```python
from build123d import *

# Parameters (mm, degrees)
SKETCH1_W               = 20
SKETCH1_H               = 20
BOSS_EXTRUDE1_DEPTH     = 20
CUT_EXTRUDE1_DEPTH      = 1
CUT_EXTRUDE1_DEPTH_BACK = 21
SKETCH3_R               = 3
CUT_EXTRUDE2_DEPTH      = 21
SKETCH4_R               = 3
CUT_EXTRUDE3_DEPTH      = 21
SKETCH5_W               = 15
SKETCH5_H               = 15
CUT_EXTRUDE5_DEPTH      = 17.5
FILLET1_R               = 0.5


with BuildPart() as part:
    # Sketch1 → Boss-Extrude1 (new body)
    with BuildSketch(Plane(origin=(0, 0, 0), x_dir=(1, 0, 0), z_dir=(0, 1, 0))):
        Rectangle(SKETCH1_W, SKETCH1_H)
    extrude(amount=BOSS_EXTRUDE1_DEPTH)

    # Sketch2 → Cut-Extrude1 (cut, two sides)
    with BuildSketch(Plane.XY.offset(10)) as cut_extrude1_sk:
        Polygon((-10, 0), (10, 20), (-10, 20), align=None)
    extrude(amount=CUT_EXTRUDE1_DEPTH, mode=Mode.SUBTRACT)
    extrude(cut_extrude1_sk.sketch, amount=-CUT_EXTRUDE1_DEPTH_BACK, mode=Mode.SUBTRACT)

    # Sketch3 → Cut-Extrude2 (cut, through all)
    with BuildSketch(Plane(origin=(10, 0, 0), x_dir=(0, 0, -1), z_dir=(1, 0, 0))):
        with Locations((0, 10)):
            Circle(SKETCH3_R)
    extrude(amount=-CUT_EXTRUDE2_DEPTH, mode=Mode.SUBTRACT)

    # Sketch4 → Cut-Extrude3 (cut, through all)
    with BuildSketch(Plane.XZ):
        Circle(SKETCH4_R)
    extrude(amount=-CUT_EXTRUDE3_DEPTH, mode=Mode.SUBTRACT)

    # Sketch5 → Cut-Extrude5 (cut)
    with BuildSketch(Plane(origin=(0, 20, 0), x_dir=(1, 0, 0), z_dir=(0, 1, 0))):
        Rectangle(SKETCH5_W, SKETCH5_H)
    extrude(amount=-CUT_EXTRUDE5_DEPTH, mode=Mode.SUBTRACT)

    # Fillet1
    fillet1_edges = [part.edges().sort_by_distance(p)[0] for p in [
        (10, 20, 0),
        (-10, 0, 0),
        (10, 0, 0),
    ]]
    fillet(fillet1_edges, radius=FILLET1_R)


solid = part.part
```
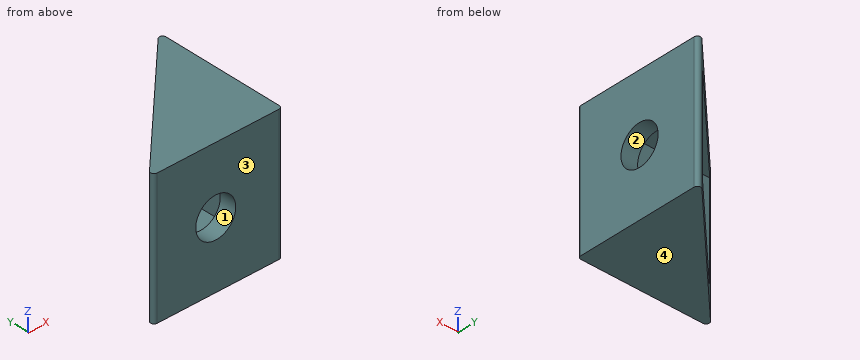
Read the model definition and answer for the solid it produces. Units are mm, in the model's axes. Face numbers are marked on the shaded views. Coordinates: 2 decimals unless noted, no trailing zeros. Write each loop counter-clockwise with the first axis right and the second up, starting at its lowest first coordinate (ties: lowest second). Pieces come first, ordered by that corner, then holes. Notation, with made-up numbers: (43, 74) -> (52, 74) arc R29 ccw to (52, 94) -> close; hole circle Ø4 at (72, 63). An arc over 180 degrees is marked (long way). Answer as a JSON object with one key per item and string values.
Q1. The part is cut by section B-B on z = 0. Give the vertices of the cut face in (x, y), then the cut area to 3 significant figures.
The answers:
{"outline": "(-9.15, 0.85) arc R0.5 ccw to (-8.79, 0) -> (-3, 0) -> (-3, 2.5) -> (-7.5, 2.5) -> close; (3, 0) -> (9.5, 0) arc R0.5 ccw to (10, 0.5) -> (10, 7) -> (7.5, 7) -> (7.5, 2.5) -> (3, 2.5) -> close; (7.5, 13) -> (10, 13) -> (10, 18.79) arc R0.5 ccw to (9.15, 19.15) -> (7.5, 17.5) -> close", "area": "56.8 mm2"}
Q2. The part is cut by section C-C on y = 10. Give the vertices of the cut face in (x, z).
The answers:
{"outline": "(0, -10) -> (10, -10) -> (10, -3) -> (7.5, -3) -> (7.5, -7.5) -> (0, -7.5) -> close; (0, 7.5) -> (7.5, 7.5) -> (7.5, 3) -> (10, 3) -> (10, 10) -> (0, 10) -> close"}
Q3. Determine the mould class of the marked faces 1, 2, 3 and 4 for opening direction Z: pulls with the +Z half, pulls with the -Z half, needs draft (parallel to the pull), parting line crosses it, or undercut.
The answers:
{"face 1": "undercut", "face 2": "undercut", "face 3": "needs draft", "face 4": "pulls with the -Z half"}
Q4. Flat-ended cylindrical pins translate along their axes: pin 1 Ø4 at (x, z) = (5, 5) entering from +Y; pin 2 Ø4 at (y, z) = (11, 2) entering from -X. Find the tip coordinate at first contact, or state that the pin passes through.
The answers:
{"pin 1": "stops at y = 2.5", "pin 2": "stops at x = 7.5"}
Q5. The part is cut by section A-A on x = 0. Give the vertices of the cut face in (y, z), then the cut area to 3 significant figures.
The answers:
{"outline": "(0, -10) -> (10, -10) -> (10, -7.5) -> (2.5, -7.5) -> (2.5, -3) -> (0, -3) -> close; (0, 3) -> (2.5, 3) -> (2.5, 7.5) -> (10, 7.5) -> (10, 10) -> (0, 10) -> close", "area": "72.5 mm2"}
Q6. The part is cut by section D-D on y = 5.5. Give the vertices of the cut face in (x, z).
The answers:
{"outline": "(-4.5, -10) -> (10, -10) -> (10, 10) -> (-4.5, 10) -> (-4.5, 7.5) -> (7.5, 7.5) -> (7.5, -7.5) -> (-4.5, -7.5) -> close"}
Q7. Consider line 1 (Z direction, x = 6.5, y = 5.75); line 2 (Y direction, x = 2.5, z = -2.5); line 3 (Y direction, x = 8.65, z = 0). Determine where each line is inside the solid, lowest interval first. Write a range as [from, to].
The answers:
{"line 1": "z = [-10, -7.5], [7.5, 10]", "line 2": "y = [0, 2.5]", "line 3": "y = [0, 7], [13, 18.65]"}
